```python
from build123d import *

# Parameters (mm, degrees)
SKETCH1_W            = 60
SKETCH1_H            = 58
BOSS_EXTRUDE1_DEPTH  = 7
M4_CLEARANCE_HOLE2_D = 4.5
LPATTERN1_COUNT      = 2
LPATTERN1_PITCH      = 13
M4_CLEARANCE_HOLE4_D = 4.5
CUT_EXTRUDE5_DEPTH   = 84.743656476
FILLET3_R            = 10


with BuildPart() as part:
    # Sketch1 → Boss-Extrude1 (new body)
    with BuildSketch(Plane(origin=(0, 0, 0), x_dir=(1, 0, 0), z_dir=(0, 1, 0))):
        with Locations((30, 29)):
            Rectangle(SKETCH1_W, SKETCH1_H)
    extrude(amount=BOSS_EXTRUDE1_DEPTH)

    # M4 Clearance Hole2 (through all)
    with Locations(Plane(origin=(0, 0, 0), x_dir=(-1, 0, 0), z_dir=(0, -1, 0))):
        with Locations((-25, 36.5), (-25, 21.5)):
            m4_clearance_hole2 = Hole(M4_CLEARANCE_HOLE2_D / 2)

    # LPattern1: M4 Clearance Hole2 ×2
    with Locations(*[(i * LPATTERN1_PITCH, 0, 0) for i in range(1, LPATTERN1_COUNT)]):
        add(m4_clearance_hole2, mode=Mode.SUBTRACT)

    # M4 Clearance Hole4 (through all)
    with Locations(Plane(origin=(0, 0, 0), x_dir=(-1, 0, 0), z_dir=(0, -1, 0))):
        with Locations((-50, 49), (-50, 9), (-10, 29)):
            Hole(M4_CLEARANCE_HOLE4_D / 2)

    # Sketch29 → Cut-Extrude5 (cut, through all)
    with BuildSketch(Plane.XZ):
        Polygon((40, 0), (28, -12), (14, -12), (0, -26), (0, 0), align=None)
        Polygon((0, -32), (0, -58), (40, -58), (28, -46), (14, -46), align=None)
    extrude(amount=-CUT_EXTRUDE5_DEPTH, mode=Mode.SUBTRACT)

    # Fillet3
    # the kernel refuses this fillet: 10 mm, written as the material it adds along each edge
    with BuildSketch(Plane(origin=(28, 0, -46), x_dir=(-1, 0, 0), z_dir=(0, 1, 0)), Plane(origin=(28, 0, -12), x_dir=(0.7071067811865417, 0, 0.7071067811865532), z_dir=(0, 1, 0))) as fillet3_piece_1:
        with BuildLine():
            CenterArc((FILLET3_R * 0.414213562373, -FILLET3_R), FILLET3_R, 90, 45)
            Line((-FILLET3_R * 0.292893218813, -FILLET3_R * 0.292893218813), (0, 0))
            Line((0, 0), (FILLET3_R * 0.414213562373, 0))
        make_face()
    extrude(amount=7)
    # the kernel refuses this fillet: 10 mm, written as the material it takes off along each edge
    with BuildSketch(Plane(origin=(60, -25, 0), x_dir=(-1, 0, 0), z_dir=(0, 1, 0)), Plane(origin=(60, -25, -58), x_dir=(0, 0, 1), z_dir=(0, 1, 0))) as fillet3_2_piece_1:
        with BuildLine():
            CenterArc((FILLET3_R, -FILLET3_R), FILLET3_R, 90, 90)
            Line((0, -FILLET3_R), (0, 0))
            Line((0, 0), (FILLET3_R, 0))
        make_face()
    extrude(amount=57, mode=Mode.SUBTRACT)
    with BuildSketch(Plane(origin=(40, -10.355339059, -58), x_dir=(-0.7071067811865415, 0, 0.7071067811865536), z_dir=(0, 1, 0)), Plane(origin=(14, -10.355339059, -46), x_dir=(-0.7071067811865411, 0, 0.707106781186554), z_dir=(0, 1, 0)), Plane(origin=(0, -10.355339059, -32), x_dir=(0, 0, 1), z_dir=(0, 1, 0)), Plane(origin=(0, -10.355339059, -26), x_dir=(0.7071067811865417, 0, 0.7071067811865532), z_dir=(0, 1, 0)), Plane(origin=(14, -10.355339059, -12), x_dir=(1, 0, 0), z_dir=(0, 1, 0)), Plane(origin=(40, -10.355339059, 0), x_dir=(1, 0, 0), z_dir=(0, 1, 0))) as fillet3_2_piece_2:
        with BuildLine():
            CenterArc((FILLET3_R * 0.414213562373, FILLET3_R), FILLET3_R, 225, 45)
            Line((-FILLET3_R * 0.292893218813, FILLET3_R * 0.292893218813), (0, 0))
            Line((0, 0), (FILLET3_R * 0.414213562373, 0))
        make_face()
    extrude(amount=27.710678119, mode=Mode.SUBTRACT)


solid = part.part
```
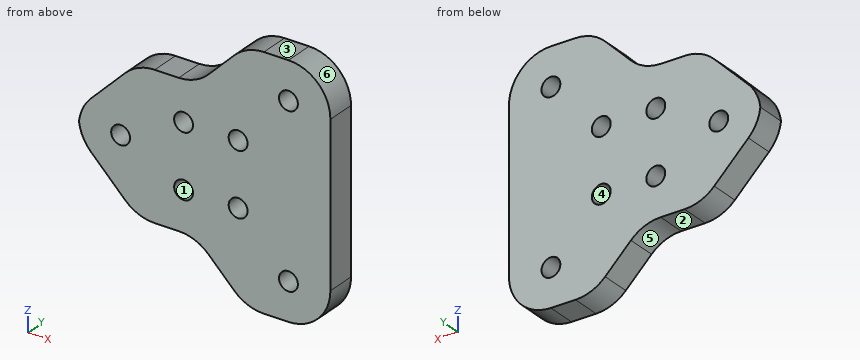
Verification items for the finished model (mm, model axes). Face numbers are marked on the shaded views. A direction names the side the tool comes from. Round coordinates to 2 decimals unless told otherwise and drop trailing zeros. Write each loop counter-clockwise with the first axis right and the second up, starting at its lowest first coordinate (ties: lowest second). Pieces come first, ordered by that corner, then holes. Notation, with made-up numbers: (44.25, -36) -> (59.25, -36) arc R26 cw to (59.25, -16) -> close; hole circle Ø6 at (-37, 27.25). An arc over 180 degrees is marked (long way). Write each question's results on one line, items separated by ' | '. Start each with the question number.
1. Cross-section at B-B (z = -36.5). Enter the section's corners in (x, y), then the cut area to 4 significant figures.
2. Cross-section at A-A (y = 1.75). Enter the section's corners in (x, z).
3. Cross-section at C-C (x = 9.5). Enter the section's corners in (y, z).
4. Set-up check for the marked faces 1 and 2: record each of +Z, -Z, +X, -X, +Y, -Y from which the full face is reachable in a straight line by a thin tool's end or side.
5. Depth check by flat-ended pin: P1, Ø4, axis at x = 50, z = -49, coming from the +Y side; P2, Ø3, axis at x = 29, y = 2, coming from the -Z side; P3, Ø4, axis at x = 22.5, y = 0.5, coming from the -Z side; P4, Ø6, axis at x = 38, z = -36.5, coming from the -Y side. Enter the tip coordinate at first touch or a pass-through.
6. Material ranges on probe 1 along Z at (x, y) = (50, 4.25); probe 2 along X at (y, z) = (1.5, -21); probe 3 along X at (y, z) = (2.5, -36.5), recorded low to high. Write a range as from..to.
7. Draft check along X on the marked faces 3, 4, 5 and 6. Enter one of: +X half, -X half, draft (parallel to the pull), parting line (faces both ways), or undercut.
8. Cross-section at D-D (x = 38). Enter the section's corners in (y, z), then the cut area to 3 significant figures.
Solutions:
1) outline: (4.5, 0) -> (22.75, 0) -> (22.75, 7) -> (4.5, 7) -> close; (27.25, 0) -> (35.75, 0) -> (35.75, 7) -> (27.25, 7) -> close; (40.25, 0) -> (60, 0) -> (60, 7) -> (40.25, 7) -> close | area: 325.5 mm2
2) outline: (0.07, -29) arc R10 ccw to (2.93, -34.93) -> (11.07, -43.07) arc R10 ccw to (18.14, -46) -> (23.86, -46) arc R10 cw to (30.93, -48.93) -> (37.07, -55.07) arc R10 ccw to (44.14, -58) -> (50, -58) arc R10 ccw to (60, -48) -> (60, -10) arc R10 ccw to (50, 0) -> (44.14, 0) arc R10 ccw to (37.07, -2.93) -> (30.93, -9.07) arc R10 cw to (23.86, -12) -> (18.14, -12) arc R10 ccw to (11.07, -14.93) -> (2.93, -23.07) arc R10 ccw to start; hole circle Ø4.5 at (10, -29); hole circle Ø4.5 at (25, -36.5); hole circle Ø4.5 at (25, -21.5); hole circle Ø4.5 at (38, -36.5); hole circle Ø4.5 at (38, -21.5); hole circle Ø4.5 at (50, -49); hole circle Ø4.5 at (50, -9)
3) outline: (0, -41.5) -> (7, -41.5) -> (7, -31.19) -> (0, -31.19) -> close; (0, -26.81) -> (7, -26.81) -> (7, -16.5) -> (0, -16.5) -> close
4) face 1: +Y, -Y | face 2: -Z, -X, +Y, -Y
5) P1: passes through | P2: stops at z = -48.52 | P3: stops at z = -46.02 | P4: stops at y = 0
6) probe 1: z = -58..-51.25, -46.75..-11.25, -6.75..0 | probe 2: x = 5..22.81, 27.19..35.81, 40.19..60 | probe 3: x = 4.5..22.75, 27.25..35.75, 40.25..60
7) face 3: draft | face 4: undercut | face 5: -X half | face 6: +X half
8) outline: (0, -55.89) -> (7, -55.89) -> (7, -38.75) -> (0, -38.75) -> close; (0, -34.25) -> (7, -34.25) -> (7, -23.75) -> (0, -23.75) -> close; (0, -19.25) -> (7, -19.25) -> (7, -2.11) -> (0, -2.11) -> close | area: 313 mm2
